from build123d import *

# Parameters (mm, degrees)
SKETCH1_W           = 77.202171331
SKETCH1_H           = 55.481682761
BOSS_EXTRUDE1_DEPTH = 5
SKETCH2_W           = 4.968888078
SKETCH2_H           = 55.481682761
BOSS_EXTRUDE2_DEPTH = 67.858
SKETCH3_R           = 4.957767387
SKETCH3_R_2         = 4.980451749
CUT_EXTRUDE1_DEPTH  = 67.858
SKETCH4_R           = 5.025637378
SKETCH4_R_2         = 5.040484197
CUT_EXTRUDE2_DEPTH  = 67.858
FILLET1_R           = 10
FILLET2_R           = 2
FILLET3_R           = 1


with BuildPart() as part:
    # Sketch1 → Boss-Extrude1 (new body)
    with BuildSketch(Plane(origin=(0, 0, 0), x_dir=(1, 0, 0), z_dir=(0, 1, 0))):
        with Locations((38.601085666, 27.740841381)):
            Rectangle(SKETCH1_W, SKETCH1_H)
    extrude(amount=BOSS_EXTRUDE1_DEPTH)

    # Sketch2 → Boss-Extrude2 (add)
    with BuildSketch(Plane(origin=(0, 5, 0), x_dir=(1, 0, 0), z_dir=(0, 1, 0))):
        with Locations((2.484444039, 27.740841381)):
            Rectangle(SKETCH2_W, SKETCH2_H)
    extrude(amount=BOSS_EXTRUDE2_DEPTH)

    # Sketch3 → Cut-Extrude1 (cut)
    with BuildSketch(Plane(origin=(0, 5, 0), x_dir=(1, 0, 0), z_dir=(0, 1, 0))):
        with Locations((63.211940842, 41.114585833)):
            Circle(SKETCH3_R)
        with Locations((63.211940842, 15.158442754)):
            Circle(SKETCH3_R_2)
    extrude(amount=-CUT_EXTRUDE1_DEPTH, mode=Mode.SUBTRACT)

    # Sketch4 → Cut-Extrude2 (cut)
    with BuildSketch(Plane(origin=(4.968888078, 0, 0), x_dir=(0, 0, -1), z_dir=(1, 0, 0))):
        with Locations((14.790160446, 55.661727657)):
            Circle(SKETCH4_R)
        with Locations((39.821700462, 55.661727657)):
            Circle(SKETCH4_R_2)
    extrude(amount=-CUT_EXTRUDE2_DEPTH, mode=Mode.SUBTRACT)

    # Fillet1
    fillet1_edges = [part.edges().sort_by_distance(p)[0] for p in [
        (4.968888078, 5, -27.74084138),
    ]]
    fillet(fillet1_edges, radius=FILLET1_R)

    # Fillet2
    fillet2_edges = [part.edges().sort_by_distance(p)[0] for p in [
        (4.968888078, 72.858, -27.74084138),
        (4.968888078, 43.929, -55.481682761),
        (7.897820266, 7.928932188, -55.481682761),
        (46.085529705, 5, -55.481682761),
        (77.202171331, 5, -27.74084138),
        (46.085529705, 5, 0),
        (7.897820266, 7.928932188, 0),
        (4.968888078, 43.929, 0),
    ]]
    fillet(fillet2_edges, radius=FILLET2_R)

    # Fillet3
    fillet3_edges = [part.edges().sort_by_distance(p)[0] for p in [
        (58.254173454, 5, -41.114585833),
        (58.231489093, 5, -15.158442754),
        (4.968888078, 55.661727657, -9.764523068),
        (4.968888078, 55.661727657, -34.781216265),
    ]]
    fillet(fillet3_edges, radius=FILLET3_R)


solid = part.part
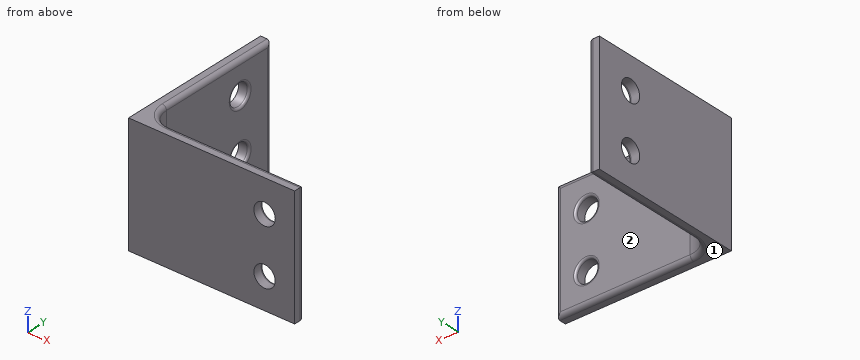
Input: part model. Units: mm. Frame: model coordinates. Face numbers are marked on the shaded views. A direction names the side the tool comes from. Coordinates: 2 decimals unless noted, no trailing zeros. Loops run counter-clockwise (first coordinate to the right, second up) from the corner with the lowest first, then second, coordinate; pieces in that order, holes last.
Q1. Cut plane B-B (x = 19). Output: boundary loops of the cut face in (y, z), then the cut area to 3 significant figures.
Q2. Material intervals for line 1 (X direction, y = 17.5, z = -13); line 2 (Y direction, x = 64, z = -3), sorted ascending.
Q3. Cut plane D-D (z = -39.5). Give the number of separate pieces and of enclosed holes in the cut face, then the cut area to 3 significant figures.
Q4. Cut plane C-C (y = 30). Output: boundary loops of the cut face in (x, z), then the cut area to 3 significant figures.
Q5. Cut plane A-A (z = -7). Output: boundary loops of the cut face in (x, y), then the cut area to 3 significant figures.
Q6. Set-up query: the marked faces 1 and 2. Return all of +Z, -Z, +X, -X, +Y, -Y with unobstructed straight access to the full face (end or side cutting, diameter ignored); none if empty.
Q7. Contact query for flat-ended pins moving along their axis: pin 1 (13 mm diameter, centred on y = 55.66, z = -14.79, fed in from +X); pin 2 (13 mm diameter, centred on y = 55.66, z = -39.82, fed in from -X); pin 3 (1.5 mm diameter, centred on x = 54.5, z = -35.5, fed in from +Y). Output: stop coordinate, or through.
Working result:
1. outline: (0, -55.48) - (3, -55.48) arc R2 ccw to (5, -53.48) - (5, -2) arc R2 ccw to (3, 0) - (0, 0) - close
1. area: 276 mm2
2. line 1: x = 0 to 4.97
2. line 2: y = 0 to 5
3. separate pieces: 3
3. enclosed holes: 0
3. area: 645 mm2
4. outline: (0, -55.48) - (2.97, -55.48) arc R2 ccw to (4.97, -53.48) - (4.97, -2) arc R2 ccw to (2.97, 0) - (0, 0) - close
4. area: 274 mm2
5. outline: (0, 0) - (77.2, 0) - (77.2, 3) arc R2 ccw to (75.2, 5) - (14.97, 5) arc R10 cw to (4.97, 15) - (4.97, 70.86) arc R2 ccw to (2.97, 72.86) - (0, 72.86) - close
5. area: 743 mm2
6. face 1: -Z, +X, -X, +Y, -Y
6. face 2: +Z, -Z, +X, +Y
7. pin 1: stops at x = 4.97
7. pin 2: stops at x = 0
7. pin 3: stops at y = 5
